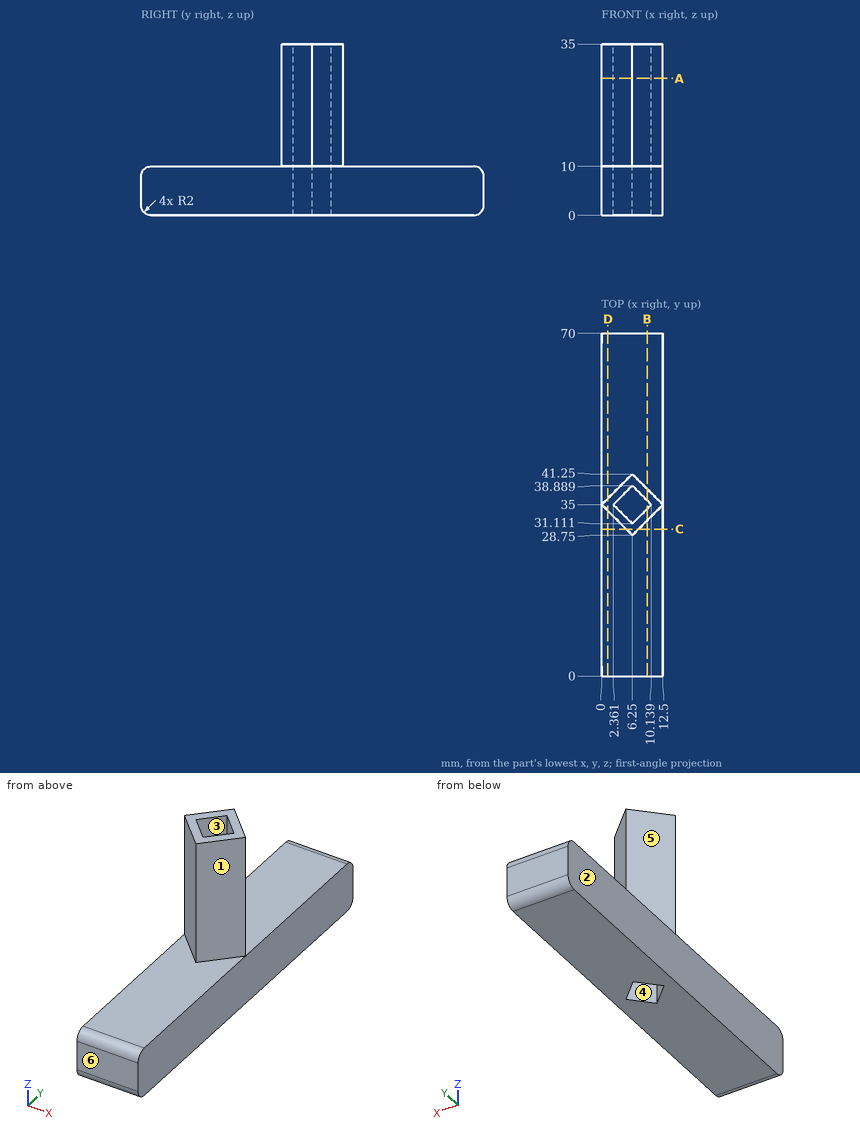
Source: three-view drawing plus pictorial views. Frame: mm from the lowest corner of the part. A direction names the side the tool comes from. Round coordinates to 2 decimals unless told otherwise and drop trailing zeros. Loops run counter-clockwise (first coordinate to the right, second up) from the corner with the lowest first, then second, coordinate; pieces in that order, holes last. Notation, with made-up numbers: M -17,62.25 L 26,62.25 A33 cw 26,93.25 Z; hole C -29.5,57.5 d10. An arc over 180 degrees is marked long. Answer as CSV lines item,"result".
Q1. Cut plane A-A (z = 28). Return the cut outline in (x, y), plus the area to 3 significant figures.
Verdict:
outline,"M 0,35 L 6.25,28.75 L 12.5,35 L 6.25,41.25 Z; hole M 2.36,35 L 6.25,31.11 L 10.14,35 L 6.25,38.89 Z"
area,"47.9 mm^2"
Q2. Reachability of the marked faces 4, 5 and 6 from +Z, -Z, +X, -X, +Y, -Y: full face, straight path, thin tool, end or side. Return the list, or none.
Verdict:
face 4,"+Z, -Z"
face 5,"+Z, -X, +Y"
face 6,"+Z, -Z, +X, -X, -Y"
Q3. Cut plane B-B (x = 9.25). Return the cut outline in (y, z), plus the area to 3 significant figures.
Verdict:
outline,"M 0,2 A2 ccw 2,0 L 34.11,0 L 34.11,35 L 31.75,35 L 31.75,10 L 2,10 A2 ccw 0,8 Z; M 35.89,0 L 68,0 A2 ccw 70,2 L 70,8 A2 ccw 68,10 L 38.25,10 L 38.25,35 L 35.89,35 Z"
area,"797 mm^2"
Q4. Cut plane C-C (y = 30). Return the cut outline in (x, z).
Verdict:
outline,"M 0,0 L 12.5,0 L 12.5,10 L 7.5,10 L 7.5,35 L 5,35 L 5,10 L 0,10 Z"
Q5. Contact query for flat-ended pins moving along their axis: pin 1 (3 mm diameter, centred on x = 9, z = 21, fed in from +Y); pin 2 (4 mm diameter, centred on x = 3.5, y = 20.5, fed in from +Z). Output: stop coordinate, or through.
Verdict:
pin 1,"stops at y = 40"
pin 2,"stops at z = 10"
Q6. Cut plane D-D (x = 1.25). Return the cut outline in (y, z).
Verdict:
outline,"M 0,2 A2 ccw 2,0 L 68,0 A2 ccw 70,2 L 70,8 A2 ccw 68,10 L 36.25,10 L 36.25,35 L 33.75,35 L 33.75,10 L 2,10 A2 ccw 0,8 Z"
Q7. Line query: line 1 along Z through (x, y) = (2.25, 60); line 2 along Y through (x, z) = (9.5, 4); line 3 along Y through (x, z) = (9.25, 11). Output: solid intervals per line, ascending.
Verdict:
line 1,"z = 0 to 10"
line 2,"y = 0 to 34.36, 35.64 to 70"
line 3,"y = 31.75 to 34.11, 35.89 to 38.25"
Q8. Pull-direction query (Y, two-part tool) for the marked faces 1, 2 and 3; classes: +Y half, -Y half, draft (parallel to the pull), parting line (faces both ways), or undercut.
Verdict:
face 1,"-Y half"
face 2,"draft"
face 3,"undercut"
